Study the drawing (mm; zero at the part's minimum x, y, z) and answer. A direction names the side the tool comes from. Give positions to 0.01 mm unless a question says otherwise; leave off trailing zeros. Write each loop counter-clockwise with the first axis right and the second up, starting at its lowest first coordinate (ties: lowest second). Pieces come first, ordered by that corner, then holes. Notation, with made-up numbers: (77.25, 60.5) - (130.25, 60.5) arc R13 ccw to (130.25, 68.5) - close; hole circle Ø1 at (15.5, 46). An arc over 180 degrees is marked (long way). Answer in a Markdown table with one row per item. Add a question column.
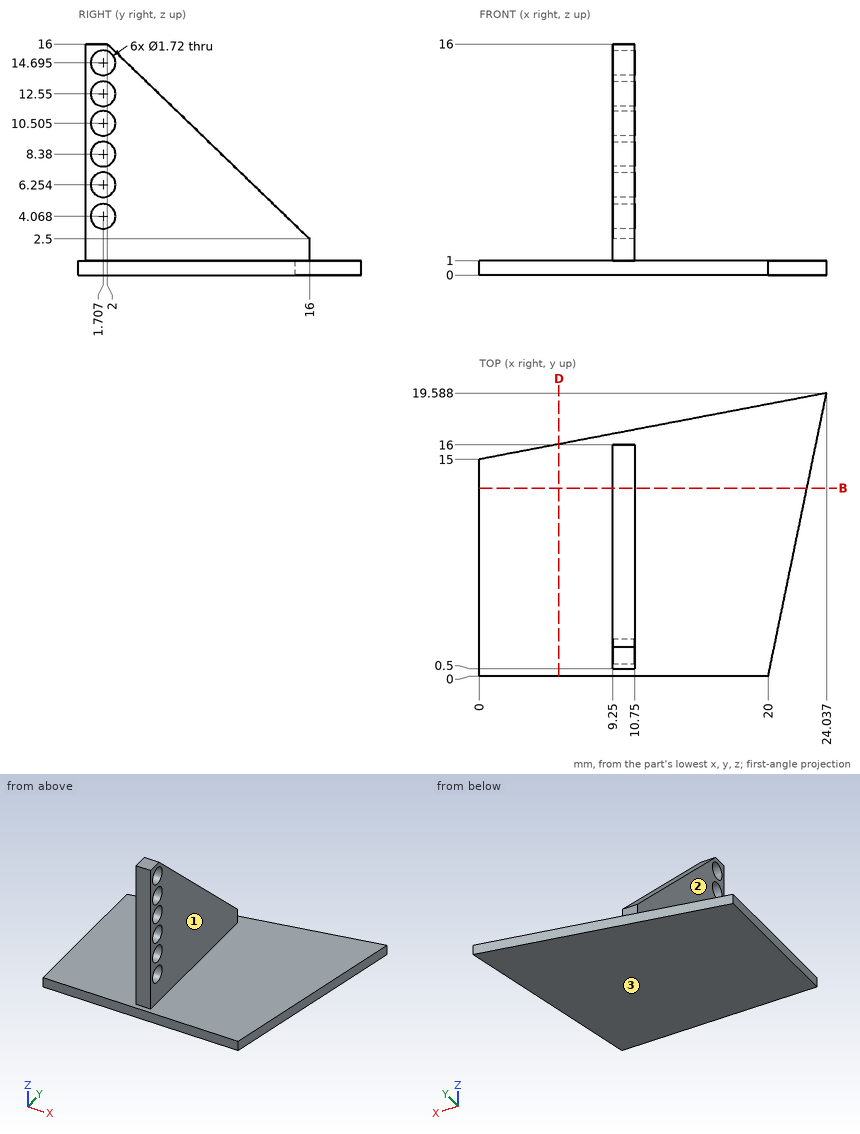
1. Section D-D (x = 5.5) is taken. Give the vertices of the cut face in (y, z).
2. Straight lines are drawn through the part: L1, parallel to Z at x = 2.25, y = 2; L2, parallel to Y at x = 9.5, z = 5 (1 decimal); L3, parallel to X at y = 4.25, z = 9. For each, find the intervals that lie inside material, in ascending order. Write a range as [from, to].
3. A tool of negligible diameter and unlimited length cuts with its end or side. For the marked faces 1, 2 and 3, from which of +Z, -Z, +X, -X, +Y, -Y can it reach the whole face along a straight path? Write none if from no direction.
4. Section B-B (y = 13) is taken. Give the vertices of the cut face in (x, z).
5. Given pin 1 Ø3 at (y, z) = (13, 3.5) entering from -X; pin 2 Ø6 at (x, y) = (19, 15.5) entering from +Z; pin 3 Ø3 at (y, z) = (1.71, 14.7) entering from +X; pin 4 Ø1.4 at (y, z) = (1.71, 12.55) entering from -X, each flat-ended and moving along its own axis, determine where each tip first touches the part or whether it passes through.
Geometry check:
| question | item | result |
|---|---|---|
| 1 | outline | (0, 0) - (16.05, 0) - (16.05, 1) - (0, 1) - close |
| 2 | L1 | [0, 1] |
| 2 | L2 | [0.5, 13.4] |
| 2 | L3 | [9.25, 10.75] |
| 3 | face 1 | +Z, +X, +Y, -Y |
| 3 | face 2 | +Z, -X, +Y, -Y |
| 3 | face 3 | -Z, +X, -X, +Y, -Y |
| 4 | outline | (0, 0) - (22.68, 0) - (22.68, 1) - (10.75, 1) - (10.75, 5.39) - (9.25, 5.39) - (9.25, 1) - (0, 1) - close |
| 5 | pin 1 | x = 9.25 |
| 5 | pin 2 | z = 1 |
| 5 | pin 3 | x = 10.75 |
| 5 | pin 4 | through |
